Verification items for this drawing (mm, ordinates from the low corner). Round coordinates to 2 decimals unless told otherwise and drop trailing zeros. Order: outer loops, then holes, each group sorted by start corner. A loop starts at its lowest first (then second) coordinate and runs counter-clockwise, first axis right, second up. Notation, with made-up numbers: M 75,71.25 L 89,71.25 A21 ccw 89,82.25 Z; hole C 59.5,-3 d11. An arc over 180 degrees is marked long. One line per item, written item: value. Start each with the question number.
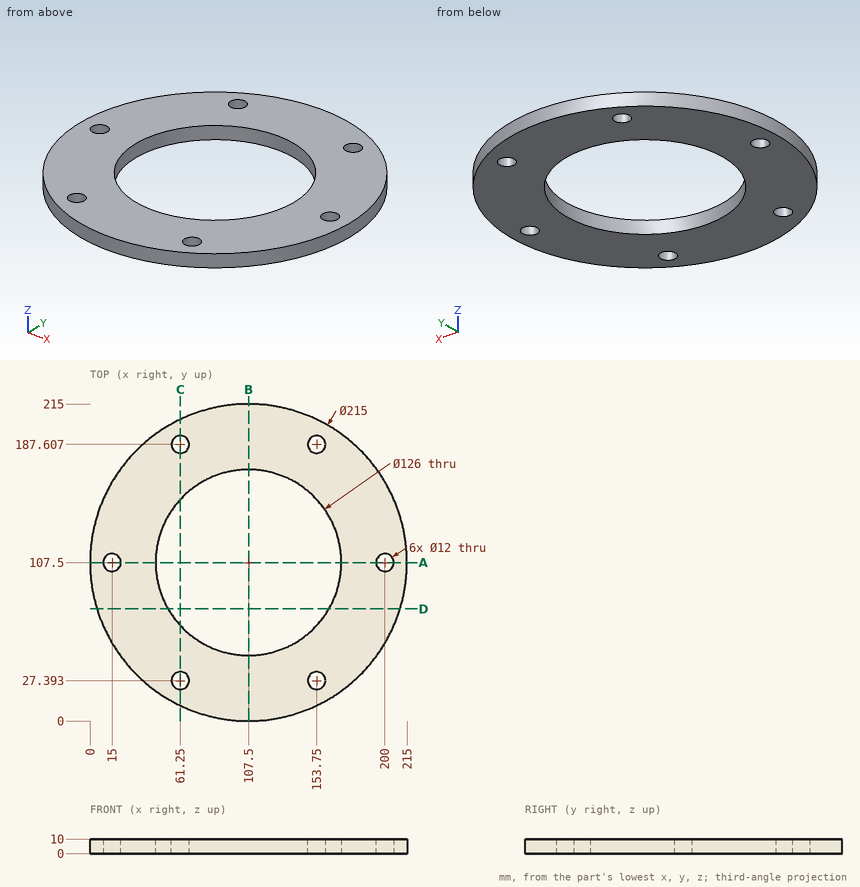
1. Scan lines: line 1 along X through (y, z) = (30, 8.25) (1 decimal); line 2 along Y through (x, z) = (150, 8.25) (1 decimal); line 3 along Y through (x, z) = (153.75, 5.75). Record each from-to range of solid material in increasing order.
2. Section check A-A (y = 107.5). Record the cut outline in (x, z).
3. Section check D-D (y = 76). Record the cut outline in (x, z).
4. Section check C-C (x = 61.25). Record the cut outline in (y, z), and give its area (3 significant figures).
5. Section check B-B (x = 107.5). Record the cut outline in (y, z).
6. Depth check by flat-ended pin: pin 1 (3 mm diameter, centred on y = 169.5, z = 4.5, fed in from -X); pin 2 (4 mm diameter, centred on y = 133.5, z = 7, fed in from +X); pin 3 (6 mm diameter, centred on x = 68.5, y = 60, fed in from +Z); pin 4 (11 mm diameter, centred on x = 153.75, y = 187.61, fed in from +Z). Enter the tip coordinate at first touch or a pass-through.
Geometry check:
1. line 1: x = 33 to 55.8, 66.7 to 148.3, 159.2 to 182
1. line 2: y = 8.8 to 22.7, 32.1 to 61, 154 to 182.9, 192.3 to 206.2
1. line 3: y = 10.46 to 21.39, 33.39 to 64.72, 150.28 to 181.61, 193.61 to 204.54
2. outline: M 0,0 L 9,0 L 9,10 L 0,10 Z; M 21,0 L 44.5,0 L 44.5,10 L 21,10 Z; M 170.5,0 L 194,0 L 194,10 L 170.5,10 Z; M 206,0 L 215,0 L 215,10 L 206,10 Z
3. outline: M 4.72,0 L 52.94,0 L 52.94,10 L 4.72,10 Z; M 162.06,0 L 210.28,0 L 210.28,10 L 162.06,10 Z
4. outline: M 10.46,0 L 21.39,0 L 21.39,10 L 10.46,10 Z; M 33.39,0 L 64.72,0 L 64.72,10 L 33.39,10 Z; M 150.28,0 L 181.61,0 L 181.61,10 L 150.28,10 Z; M 193.61,0 L 204.54,0 L 204.54,10 L 193.61,10 Z
4. area: 845 mm²
5. outline: M 0,0 L 44.5,0 L 44.5,10 L 0,10 Z; M 170.5,0 L 215,0 L 215,10 L 170.5,10 Z
6. pin 1: stops at x = 18.64
6. pin 2: stops at x = 212.29
6. pin 3: stops at z = 10
6. pin 4: passes through
